For this review, take the finished solid that the model builds, in its own axes (mm). Coordinates: 2 decimals unless noted, no trailing zeros. Order: outer loops, then holes, each group sorted by start corner. A loop starts at its lowest first (then second) coordinate and runs counter-clockwise, first axis right, second up. Notation, with made-up numbers: (86.5, 88.5) -> (99.5, 88.5) arc R29 ccw to (99.5, 121.5) -> close; hole circle Ø6 at (29.5, 26). An arc over 180 degrees is marked (long way). Return JSON: item names as keys, results as strings. Group by question number.
Item 1: Take a section at A-A (z = 2.1). Write out the cut boundary in (x, y).
Item 2: Take a section at B-B (x = -19). Write out the cut boundary in (y, z).
Item 3: Take a section at C-C (y = 0). Write out the cut boundary in (x, z), then the cut area to 3 significant figures.
Item 4: Insertion check: pin 1 (3.5 mm diameter, centred on x = 0, y = 0, fed in from +Z). The pin has a flat end and moves straight along its axis. Give the tip position at first contact, or say it passes through.
Item 5: For line 1 along Y through (x, z) = (-9, 1.05); line 2 along Y through (x, z) = (-14.5, 0.2); line 3 along X through (y, z) = (0.5, 1.35), list the stretches that pass through material, from the lowest coordinate up.
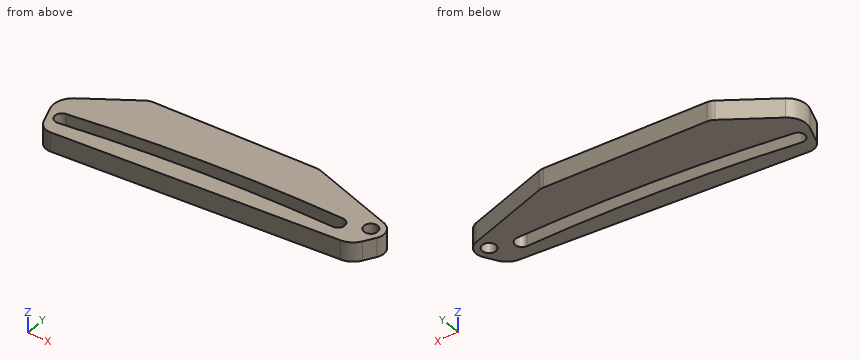
```python
from build123d import *

# Parameters (mm, degrees)
SKETCH_1_R                 = 1.05
EXTRUDE_1_DEPTH            = 3
CUT_EXTRUDE_1_DEPTH        = 3
EXTRUDE_2_DEPTH            = 3
CUT_EXTRUDE_1_2_DEPTH      = 53.507202205
CUT_EXTRUDE_1_2_DEPTH_BACK = 3
FILLET_1_R                 = 2
FILLET_2_R                 = 3
FILLET_3_R                 = 3
FILLET_4_R                 = 2


with BuildPart() as part:
    # 草图1 → 凸台-拉伸1 (new body)
    with BuildSketch(Plane.XY):
        with BuildLine():
            Line((-49.8, -9.234190916), (-51.601705413, -5.540147386))
            Line((-51.601705413, -5.540147386), (-37.679104802, 4.039580805))
            Line((-37.679104802, 4.039580805), (-12.5, 5.72552912))
            Line((-12.5, 5.72552912), (0.559507092, 1.920143696))
            ThreePointArc((0.559507092, 1.920143696), (1.855968535, 0.745238752), (1.732050808, -1))
            Line((1.732050808, -1), (0, -4))
            Line((0, -4), (-49.8, -9.234190916))
        make_face()
        Circle(SKETCH_1_R, mode=Mode.SUBTRACT)
    extrude(amount=EXTRUDE_1_DEPTH)

    # 草图3 → Cut-Extrude 1 (cut)
    with BuildSketch(Plane.XY.offset(3)):
        with BuildLine():
            ThreePointArc((-4.02208158, -0.450232214), (-25.702985996, -1.810356042), (-47.195735426, -4.968405291))
            ThreePointArc((-47.195735426, -4.968405291), (-48.031594709, -6.195735426), (-46.804264574, -7.031594709))
            ThreePointArc((-46.804264574, -7.031594709), (-25.48441219, -3.898950185), (-3.97791842, -2.549767786))
            ThreePointArc((-3.97791842, -2.549767786), (-2.950232214, -1.47791842), (-4.02208158, -0.450232214))
        make_face()
    extrude(amount=-CUT_EXTRUDE_1_DEPTH, mode=Mode.SUBTRACT)

    # 草图5 → 凸台-拉伸2 (add)
    with BuildSketch(Plane.XY.offset(3)):
        with BuildLine():
            ThreePointArc((-44.233228768, -4.423985056), (-45.083193675, -5.64158912), (-43.865589611, -6.491554028))
            ThreePointArc((-43.865589611, -6.491554028), (-45.335706004, -6.757335859), (-46.804264574, -7.031594709))
            ThreePointArc((-46.804264574, -7.031594709), (-48.031594709, -6.195735426), (-47.195735426, -4.968405291))
            ThreePointArc((-47.195735426, -4.968405291), (-45.715267325, -4.691922292), (-44.233228768, -4.423985056))
        make_face()
    extrude(amount=-EXTRUDE_2_DEPTH)

    # 草图6 → Cut-Extrude 1 2 (cut, two sides: drawn at the far end of the back side and taken through both)
    with BuildSketch(Plane.XY.offset(3).offset(-CUT_EXTRUDE_1_2_DEPTH_BACK)):
        Polygon((-47.297047091, -2.578239778), (-44.938218964, -8.723197138), (-54.274023229, -12.306876634), (-56.632851356, -6.161919273), align=None)
    extrude(amount=CUT_EXTRUDE_1_2_DEPTH + CUT_EXTRUDE_1_2_DEPTH_BACK, mode=Mode.SUBTRACT)

    # 圆角1
    fillet_1_edges = [part.edges().sort_by_distance(p)[0] for p in [
        (-44.938218964, -8.723197138, 1.5),
    ]]
    fillet(fillet_1_edges, radius=FILLET_1_R)

    # 圆角2
    fillet_2_edges = [part.edges().sort_by_distance(p)[0] for p in [
        (0, -4, 1.5),
    ]]
    fillet(fillet_2_edges, radius=FILLET_2_R)

    # 圆角3
    fillet_3_edges = [part.edges().sort_by_distance(p)[0] for p in [
        (-47.297047091, -2.578239778, 1.5),
    ]]
    fillet(fillet_3_edges, radius=FILLET_3_R)

    # 圆角4
    fillet_4_edges = [part.edges().sort_by_distance(p)[0] for p in [
        (-12.5, 5.72552912, 1.5),
        (-37.679104802, 4.039580805, 1.5),
    ]]
    fillet(fillet_4_edges, radius=FILLET_4_R)


solid = part.part
```
Findings below:
{
 "1": {"outline": "(-46.45, -4.78) -> (-45.49, -7.29) arc R2 ccw to (-43.41, -8.56) -> (-1.52, -4.16) arc R3 ccw to (0.76, -2.68) -> (1.73, -1) arc R2 ccw to (0.56, 1.92) -> (-12.16, 5.63) arc R2 ccw to (-12.85, 5.7) -> (-37.13, 4.08) arc R2 ccw to (-38.13, 3.73) -> (-45.35, -1.24) arc R3 ccw to start; hole (-44.23, -4.42) arc R1.05 ccw to (-43.87, -6.49) arc R258.95 cw to (-3.98, -2.55) arc R1.05 ccw to (-4.02, -0.45) arc R261.05 ccw to start; hole circle Ø2.1 at (0, 0)"},
 "2": {"outline": "(-6, 0) -> (-3.3, 0) -> (-3.3, 3) -> (-6, 3) -> close; (-1.2, 0) -> (5.29, 0) -> (5.29, 3) -> (-1.2, 3) -> close"},
 "3": {"outline": "(-43.55, 0) -> (-1.05, 0) -> (-1.05, 3) -> (-43.55, 3) -> close; (1.05, 0) -> (2, 0) -> (2, 3) -> (1.05, 3) -> close", "area": "130 mm2"},
 "4": {"pin 1": "stops at z = 3"},
 "5": {"line 1": "y = -4.95 to -2.7, -0.6 to 4.71", "line 2": "y = -5.52 to -2.99, -0.88 to 5.59", "line 3": "x = -42.82 to -0.92, 0.92 to 1.94"}
}
